```python
from build123d import *

# Parameters (mm, degrees)
F0_R     = 2
F1_DEPTH = 55
F2_R     = 2.5
F3_DEPTH = 2


with BuildPart() as f1:
    # F0 (on Front) → F1 (new body)
    with BuildSketch(Plane.XZ):
        with BuildLine():
            ThreePointArc((15, 13.5), (14.56066, 14.56066), (13.5, 15))
            Line((13.5, 15), (4, 15))
            ThreePointArc((4, 15), (3.292893, 14.707107), (3, 14))
            Line((3, 14), (3, 13))
            ThreePointArc((3, 13), (3.292893, 12.292893), (4, 12))
            Line((4, 12), (7.464466, 12))
            ThreePointArc((7.464466, 12), (8.388346, 11.382683), (8.171573, 10.292893))
            Line((8.171573, 10.292893), (3.318019, 5.43934))
            ThreePointArc((3.318019, 5.43934), (2.831384, 5.114181), (2.257359, 5))
            Line((2.257359, 5), (-2.257359, 5))
            ThreePointArc((-2.257359, 5), (-2.831384, 5.114181), (-3.318019, 5.43934))
            Line((-3.318019, 5.43934), (-8.171573, 10.292893))
            ThreePointArc((-8.171573, 10.292893), (-8.388346, 11.382683), (-7.464466, 12))
            Line((-7.464466, 12), (-4, 12))
            ThreePointArc((-4, 12), (-3.292893, 12.292893), (-3, 13))
            Line((-3, 13), (-3, 14))
            ThreePointArc((-3, 14), (-3.292893, 14.707107), (-4, 15))
            Line((-4, 15), (-13.5, 15))
            ThreePointArc((-13.5, 15), (-14.56066, 14.56066), (-15, 13.5))
            Line((-15, 13.5), (-15, 4))
            ThreePointArc((-15, 4), (-14.707107, 3.292893), (-14, 3))
            Line((-14, 3), (-13, 3))
            ThreePointArc((-13, 3), (-12.292893, 3.292893), (-12, 4))
            Line((-12, 4), (-12, 7.464466))
            ThreePointArc((-12, 7.464466), (-11.382683, 8.388346), (-10.292893, 8.171573))
            Line((-10.292893, 8.171573), (-5.43934, 3.318019))
            ThreePointArc((-5.43934, 3.318019), (-5.114181, 2.831384), (-5, 2.257359))
            Line((-5, 2.257359), (-5, -2.257359))
            ThreePointArc((-5, -2.257359), (-5.114181, -2.831384), (-5.43934, -3.318019))
            Line((-5.43934, -3.318019), (-10.292893, -8.171573))
            ThreePointArc((-10.292893, -8.171573), (-11.382683, -8.388346), (-12, -7.464466))
            Line((-12, -7.464466), (-12, -4))
            ThreePointArc((-12, -4), (-12.292893, -3.292893), (-13, -3))
            Line((-13, -3), (-14, -3))
            ThreePointArc((-14, -3), (-14.707107, -3.292893), (-15, -4))
            Line((-15, -4), (-15, -13.5))
            ThreePointArc((-15, -13.5), (-14.56066, -14.56066), (-13.5, -15))
            Line((-13.5, -15), (-4, -15))
            ThreePointArc((-4, -15), (-3.292893, -14.707107), (-3, -14))
            Line((-3, -14), (-3, -13))
            ThreePointArc((-3, -13), (-3.292893, -12.292893), (-4, -12))
            Line((-4, -12), (-7.464466, -12))
            ThreePointArc((-7.464466, -12), (-8.388346, -11.382683), (-8.171573, -10.292893))
            Line((-8.171573, -10.292893), (-3.318019, -5.43934))
            ThreePointArc((-3.318019, -5.43934), (-2.831384, -5.114181), (-2.257359, -5))
            Line((-2.257359, -5), (2.257359, -5))
            ThreePointArc((2.257359, -5), (2.831384, -5.114181), (3.318019, -5.43934))
            Line((3.318019, -5.43934), (8.171573, -10.292893))
            ThreePointArc((8.171573, -10.292893), (8.388346, -11.382683), (7.464466, -12))
            Line((7.464466, -12), (4, -12))
            ThreePointArc((4, -12), (3.292893, -12.292893), (3, -13))
            Line((3, -13), (3, -14))
            ThreePointArc((3, -14), (3.292893, -14.707107), (4, -15))
            Line((4, -15), (13.5, -15))
            ThreePointArc((13.5, -15), (14.56066, -14.56066), (15, -13.5))
            Line((15, -13.5), (15, -4))
            ThreePointArc((15, -4), (14.707107, -3.292893), (14, -3))
            Line((14, -3), (13, -3))
            ThreePointArc((13, -3), (12.292893, -3.292893), (12, -4))
            Line((12, -4), (12, -7.464466))
            ThreePointArc((12, -7.464466), (11.382683, -8.388346), (10.292893, -8.171573))
            Line((10.292893, -8.171573), (5.43934, -3.318019))
            ThreePointArc((5.43934, -3.318019), (5.114181, -2.831384), (5, -2.257359))
            Line((5, -2.257359), (5, 2.257359))
            ThreePointArc((5, 2.257359), (5.114181, 2.831384), (5.43934, 3.318019))
            Line((5.43934, 3.318019), (10.292893, 8.171573))
            ThreePointArc((10.292893, 8.171573), (11.382683, 8.388346), (12, 7.464466))
            Line((12, 7.464466), (12, 4))
            ThreePointArc((12, 4), (12.292893, 3.292893), (13, 3))
            Line((13, 3), (14, 3))
            ThreePointArc((14, 3), (14.707107, 3.292893), (15, 4))
            Line((15, 4), (15, 13.5))
        make_face()
        Circle(F0_R, mode=Mode.SUBTRACT)
    extrude(amount=-F1_DEPTH)

    # F2 (on face) → F3 (cut)
    with BuildSketch(Plane.XY.offset(5)):
        with Locations((0, 12)):
            Circle(F2_R)
    extrude(amount=-F3_DEPTH, mode=Mode.SUBTRACT)


solid = f1.part
```
Check sheet for the modelled part. Datum: model origin and axes. Units: mm. A direction names the side the tool comes from. Give positions to 0.01 mm unless a question says otherwise; leave off trailing zeros. Write each loop counter-clockwise with the first axis right and the second up, starting at its lowest first coordinate (ties: lowest second). Pieces come first, ordered by that corner, then holes. Notation, with made-up numbers: (6, 75) - (62, 75) arc R18 ccw to (62, 98) - close; hole circle Ø5 at (-36, 42.25). An arc over 180 degrees is marked (long way). Answer as a JSON object with one key per item and string values. Group by question number.
1) Depth check by flat-ended pin: P1, Ø3, axis at x = 2, y = 20, coming from the -Z side; P2, Ø2.5, axis at x = 0.5, y = 40, coming from the -Z side; P3, Ø4, axis at x = 0, y = 12, coming from the +Z side. Enter the tip coordinate at first touch or a pass-through.
2) Release check for a two-part mould opening along Z. For faces 1 (the face through (-15, 27, 9)), 2 (the face through (5, 27, 0)), 3 (the face through (-9, 27, 15)) record: pulls with the +Z half, pulls with the -Z half, needs draft (parallel to the pull), parting line crosses it, or undercut.
3) Access from +Z, -Z, +X, -X, +Y, -Y to the whole of each face (thin tool, end or side, straight path). Record for faces 4 (the face through (9, 27, -15)), 5 (the face through (0, 34, 5)), 6 (the face through (12, 27, -6)).
4) Sectioned sample at A-A (z = 0). Record the cut outline in (x, y), then the cut area to 3 significant figures.
5) Thickness scan on probe 1 along Z at (x, y) = (-13, 53); probe 2 along Z at (x, y) = (0, 30). Record the ranges inside material, lowest first. Write a range as from..to.
6) Sectioned sample at B-B (x = 0). Record the cut outline in (y, z).
7) Sectioned sample at C-C (x = -6). Record the cut outline in (y, z), then the cut area to 3 significant figures.
Geometry results:
{
 "1": {"P1": "stops at z = -14.87", "P2": "stops at z = -5", "P3": "stops at z = 3"},
 "2": {"face 1": "needs draft", "face 2": "undercut", "face 3": "pulls with the +Z half"},
 "3": {"face 4": "-Z, +X, -X, +Y, -Y", "face 5": "+Z, +Y, -Y", "face 6": "+Y, -Y"},
 "4": {"outline": "(-5, 0) - (-2, 0) - (-2, 55) - (-5, 55) - close; (2, 0) - (5, 0) - (5, 55) - (2, 55) - close", "area": "330 mm^2"},
 "5": {"probe 1": "z = -15..-3, 3..15", "probe 2": "z = -5..-2, 2..5"},
 "6": {"outline": "(0, -5) - (55, -5) - (55, -2) - (0, -2) - close; (0, 2) - (55, 2) - (55, 5) - (14.5, 5) - (14.5, 3) - (9.5, 3) - (9.5, 5) - (0, 5) - close"},
 "7": {"outline": "(0, -15) - (55, -15) - (55, -12) - (0, -12) - close; (0, -8.12) - (55, -8.12) - (55, -3.88) - (0, -3.88) - close; (0, 3.88) - (55, 3.88) - (55, 8.12) - (0, 8.12) - close; (0, 12) - (55, 12) - (55, 15) - (0, 15) - close", "area": "797 mm^2"}
}
